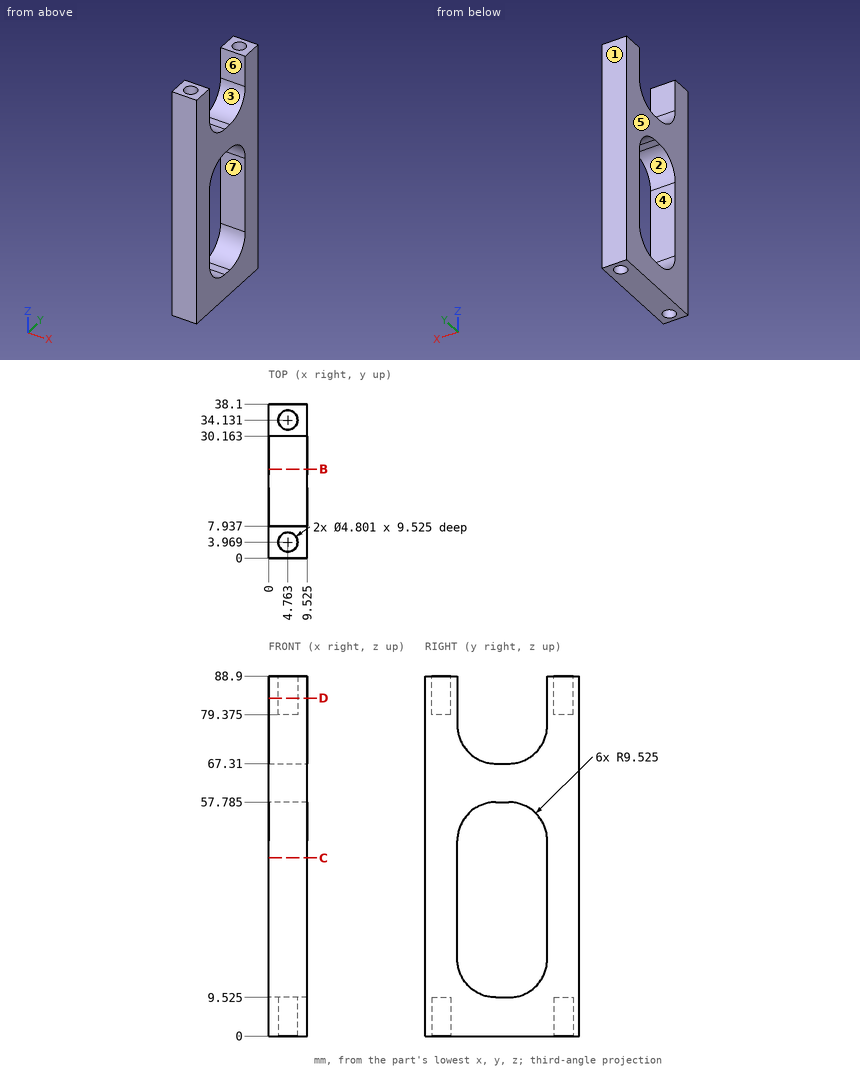
Study the drawing (mm; zero at the part's minimum x, y, z) and answer. A direction names the side the tool comes from. Round coordinates to 2 decimals unless told otherwise and drop trailing zeros. Write each loop counter-clockwise with the first axis right and the second up, starting at its lowest first coordinate (ties: lowest second). Pieces come first, ordered by that corner, then holes.
1) A cutting plane is placed at B-B on y = 22. Determine the outline of the cut face in (x, z) (1 decimal), and give its area (3 significant figures).
2) A cutting plane is placed at D-D on z = 83.5. Determine the outline of the cut face in (x, y) (1 decimal).
3) A cutting plane is placed at C-C on z = 44. Determine the outline of the cut face in (x, y) (1 decimal), and give its area (3 significant figures).
4) Consider probe 1 along Y at (x, z) = (4.75, 80); probe 2 along Y at (x, z) = (5, 47); probe 3 along Y at (x, z) = (2, 72.5). Determine where each line is inside the solid, lowest interval first.
5) Flat-ended cylindrical pins translate along their axes: P1, Ø1.4, axis at x = 4.5, y = 35, coming from the -Z side (1 decimal); P2, Ø2.5, axis at x = 4, y = 19, coming from the +Z side; P3, Ø5.5, axis at x = 5, y = 4, coming from the +Z side. Find the tip coordinate at first contact, or state that the pin passes through.
6) Which of the six approach directions +Z, -Z, +X, -X, +Y, -Y give full straight-line access (tool end or side, diameter ignored) to the marked faces 5, 6 and 7?
7) Determine the mould class of the marked faces 1, 2, 3 and 4 for opening direction Z: pulls with the +Z half, pulls with the -Z half, needs draft (parallel to the pull), parting line crosses it, or undercut.
Entries:
1. outline: (0, 0) - (9.5, 0) - (9.5, 9.6) - (0, 9.6) - close; (0, 57.7) - (9.5, 57.7) - (9.5, 67.4) - (0, 67.4) - close
1. area: 184 mm2
2. outline: (0, 0) - (9.5, 0) - (9.5, 7.9) - (0, 7.9) - close; (0, 30.2) - (9.5, 30.2) - (9.5, 38.1) - (0, 38.1) - close; hole circle Ø4.8 at (4.8, 4); hole circle Ø4.8 at (4.8, 34.1)
3. outline: (0, 0) - (9.5, 0) - (9.5, 7.9) - (0, 7.9) - close; (0, 30.2) - (9.5, 30.2) - (9.5, 38.1) - (0, 38.1) - close
3. area: 151 mm2
4. probe 1: y = 0 to 1.57, 6.37 to 7.94, 30.16 to 31.73, 36.53 to 38.1
4. probe 2: y = 0 to 7.94, 30.16 to 38.1
4. probe 3: y = 0 to 8.98, 29.12 to 38.1
5. P1: stops at z = 9.5
5. P2: stops at z = 67.31
5. P3: stops at z = 88.9
6. face 5: +Z, -Z, -X, +Y, -Y
6. face 6: +Z, +X, -X
6. face 7: +X, -X
7. face 1: needs draft
7. face 2: undercut
7. face 3: pulls with the +Z half
7. face 4: undercut
